CAD build for the part. Positions are in the model's coordinates, mm. Coordinates: 2 decimals unless noted, no trailing zeros. Order: outer loops, then holes, each group sorted by start corner. A loop starts at its lowest first (then second) coordinate and runs counter-clockwise, first axis right, second up. Notation, with made-up numbers: (-14, 30.25) - (10, 30.25) arc R33 cw to (10, 66.25) - close; hole circle Ø1 at (38.25, 44). An arc over 180 degrees is marked (long way). Use one line per item in the form item = value.
```python
from build123d import *

# Parameters (mm, degrees)
SKETCH2_W                = 33.3375
SKETCH2_H                = 12.7
CUT_EXTRUDE1_DEPTH       = 13.7
FILLET1_R                = 4
CIRPATTERN4_COUNT        = 6
FILLET1_OF_CIRPATTERN4_R = 4
SKETCH9_R                = 49.2125
SKETCH9_R_2              = 47.2125
BOSS_EXTRUDE1_DEPTH      = 12.7
SKETCH10_R               = 84.55
SKETCH10_R_2             = 82.55
BOSS_EXTRUDE2_DEPTH      = 12.7


with BuildPart() as part:
    # Sketch2 → Revolve1 (revolve)
    with BuildSketch(Plane(origin=(0, 0, 0), x_dir=(0, 0, -1), z_dir=(1, 0, 0))):
        with Locations((-65.88125, 6.35)):
            Rectangle(SKETCH2_W, SKETCH2_H)
    revolve(axis=Axis((0, -0.5, 0), (0, 1, 0)))

    # Sketch8 → Cut-Extrude1 (cut, through all)
    with BuildSketch(Plane(origin=(0, 12.7, 0), x_dir=(1, 0, 0), z_dir=(0, 1, 0))):
        with BuildLine():
            Line((-22.66059, 49.249293), (-34.364196, 69.520533))
            ThreePointArc((-34.364196, 69.520533), (0, 77.55), (34.364196, 69.520533))
            Line((34.364196, 69.520533), (22.66059, 49.249293))
            ThreePointArc((22.66059, 49.249293), (0, 54.2125), (-22.66059, 49.249293))
        make_face()
    cut_extrude1 = extrude(amount=-CUT_EXTRUDE1_DEPTH, mode=Mode.SUBTRACT)

    # Fillet1
    fillet1_edges = [part.edges().sort_by_distance(p)[0] for p in [
        (22.66059, 6.35, -49.249293),
        (-22.66059, 6.35, -49.249293),
        (-34.364196, 6.35, -69.520533),
        (34.364196, 6.35, -69.520533),
    ]]
    fillet(fillet1_edges, radius=FILLET1_R)

    # CirPattern4: Cut-Extrude1 ×6 about axis
    cirpattern4_axis = Axis((0, 0, 0), (0, 1, 0))
    for i in range(1, CIRPATTERN4_COUNT):
        add(cut_extrude1.rotate(cirpattern4_axis, i * 360 / CIRPATTERN4_COUNT), mode=Mode.SUBTRACT)

    # Fillet1 of CirPattern4
    fillet1_of_cirpattern4_edges = [part.edges().sort_by_distance(p)[0] for p in [
        (-31.320844, 6.35, -44.249293),
        (-53.981433, 6.35, -5),
        (-77.388646, 6.35, -5),
        (-43.02445, 6.35, -64.520533),
        (-53.981433, 6.35, 5),
        (-31.320844, 6.35, 44.249293),
        (-43.02445, 6.35, 64.520533),
        (-77.388646, 6.35, 5),
        (-22.66059, 6.35, 49.249293),
        (22.66059, 6.35, 49.249293),
        (34.364196, 6.35, 69.520533),
        (-34.364196, 6.35, 69.520533),
        (31.320844, 6.35, 44.249293),
        (53.981433, 6.35, 5),
        (77.388646, 6.35, 5),
        (43.02445, 6.35, 64.520533),
        (53.981433, 6.35, -5),
        (31.320844, 6.35, -44.249293),
        (43.02445, 6.35, -64.520533),
        (77.388646, 6.35, -5),
    ]]
    fillet(fillet1_of_cirpattern4_edges, radius=FILLET1_OF_CIRPATTERN4_R)

    # Sketch9 → Boss-Extrude1 (add)
    with BuildSketch(Plane(origin=(0, 0, 0), x_dir=(1, 0, 0), z_dir=(0, 1, 0))):
        Circle(SKETCH9_R)
        Circle(SKETCH9_R_2, mode=Mode.SUBTRACT)
    extrude(amount=BOSS_EXTRUDE1_DEPTH)

    # Sketch10 → Boss-Extrude2 (add)
    with BuildSketch(Plane(origin=(0, 0, 0), x_dir=(1, 0, 0), z_dir=(0, 1, 0))):
        Circle(SKETCH10_R)
        Circle(SKETCH10_R_2, mode=Mode.SUBTRACT)
    extrude(amount=BOSS_EXTRUDE2_DEPTH)


solid = part.part
```
Item 1: Cut at C-C, the plane x = -62.5. Write the cut outline in (y, z).
Derived:
outline = (0, -56.94) - (12.7, -56.94) - (12.7, -45.91) - (0, -45.91) - close; (0, -5) - (12.7, -5) - (12.7, 5) - (0, 5) - close; (0, 45.91) - (12.7, 45.91) - (12.7, 56.94) - (0, 56.94) - close
Item 2: Cut at D-D, the plane y = 9.25. State how many separate pieces and enclosed holes the cut face has, plus the area to 3 significant figures.
Derived:
separate_pieces = 1
enclosed_holes = 7
area = 7,280 mm²
Item 3: Drill centre lines: line 1 (Z direction, x = 0, y = 4.5); line 2 (Z direction, x = -8.5, y = 4.25); line 3 (X direction, y = 9, z = 0). Where is each one in solid material? Low to high. Write a range as [from, to].
Derived:
line_1 = [-84.55, -77.55], [-54.21, -47.21], [47.21, 54.21], [77.55, 84.55]
line_2 = [-84.12, -77.08], [-53.54, -46.44], [46.44, 53.54], [77.08, 84.12]
line_3 = [-84.55, -47.21], [47.21, 84.55]
Item 4: Cut at A-A, the plane x = 0. Write the cut outline in (y, z).
Derived:
outline = (0, -84.55) - (12.7, -84.55) - (12.7, -77.55) - (0, -77.55) - close; (0, -54.21) - (12.7, -54.21) - (12.7, -47.21) - (0, -47.21) - close; (0, 47.21) - (12.7, 47.21) - (12.7, 54.21) - (0, 54.21) - close; (0, 77.55) - (12.7, 77.55) - (12.7, 84.55) - (0, 84.55) - close
Item 5: Cut at B-B, the plane z = 0. Write the cut outline in (x, y), plus the area to 3 significant figures.
Derived:
outline = (-84.55, 0) - (-47.21, 0) - (-47.21, 12.7) - (-84.55, 12.7) - close; (47.21, 0) - (84.55, 0) - (84.55, 12.7) - (47.21, 12.7) - close
area = 948 mm²
Item 6: Drop flat-ended pins along their axis: pin 1 (4 mm diameter, centred on x = 68.5, y = 5.5, fed in from -Z); pin 2 (6.5 mm diameter, centred on x = -65.5, y = 7.5, fed in from +Z); pin 3 (6.5 mm diameter, centred on x = 64.5, y = 5.5, fed in from +Z) (3 decimals); pin 4 (8 mm diameter, centred on x = -63.5, z = -48.5, fed in from -Y). Give the stop position or say it passes through.
Derived:
pin_1 = -52.22
pin_2 = 57.22
pin_3 = 58.285
pin_4 = 0
Item 7: Two-plate mould, pull along Z, no slides. Class faces 1 (the face through (0.44, 6.44, 77.55)), 2 (the face through (-19, 12.7, -44)): +Z half, -Z half, draft (parallel to the pull), parting line (faces both ways), or undercut.
Derived:
face_1 = undercut
face_2 = draft
